The listing builds one solid part. Answer for the finished solid, in the listing's coordinates (mm). A direction names the side the tool comes from. Give positions to 0.01 mm unless a question says otherwise; leave off trailing zeros. Write each loop counter-clockwise with the first axis right and the second up, starting at its lowest first coordinate (ties: lowest second). Pieces come first, ordered by that corner, then holes. Notation, with made-up numbers: (30, 14.25) - (35, 14.25) arc R28 ccw to (35, 47.25) - close; hole circle Ø2 at (48.5, 51.5). An arc over 180 degrees is marked (long way). Answer as CSV lines item,"result". Start each with the question number.
(1) Straight lines are drawn through the part: probe 1 along X at (y, z) = (4, -1.5); probe 2 along Y at (x, z) = (-26, 8); probe 3 along X at (y, z) = (9.5, 3.25). For each, find the intervals that lie inside material, in ascending order.
(2) Find section C-C (z = 5.25). Write down the section's boundary in (x, y).
(3) Each of these flat-tipped pins is pushed along its axis until it touches: pin 1 Ø0.9 at (x, z) = (-18, 2) entering from -Y; pin 2 Ø6 at (x, y) = (-28, 10.5) entering from -Z; pin 3 Ø6 at (x, y) = (-21.5, 4.5) entering from +Z; pin 4 Ø8 at (x, z) = (-29.5, 10) entering from -Y. Where does it stop, or does it pass through?
(4) Find section D-D (y = 11.25). Write down the section's boundary in (x, z).
(5) Find section A-A (y = 3.5). Write down the section's boundary in (x, z).
(6) For a pull along X with two mould halves and no side action, classify faces 4 (the face through (3, 8, -1)), 5 (the face through (-53, 3, -1)), 6 (the face through (0, 6, 8)) as pulls with the +X half, pulls with the -X half, needs draft (parallel to the pull), parting line crosses it, or undercut.
(7) For faces 1 (the face through (-21, 12, -7)), 2 (the face through (-3, 5, 2)), 3 (the face through (-21, 12, 8)), determine the directions among +Z, -Z, +X, -X, +Y, -Y from which every point of the face is accessible in a straight line to the end or side of a thin tool.
(8) Find section B-B (x = -17). Write down the section's boundary in (y, z), then the cut area to 3 significant figures.
from build123d import *

# Parameters (mm, degrees)
PAD_DEPTH         = 3
PAD001_DEPTH      = 10
PAD001_DEPTH_BACK = 18
POCKET_DEPTH      = 5


with BuildPart() as part:
    # Sketch → Pad (new body)
    with BuildSketch(Plane.XY):
        Polygon((-43, 12), (0, 12), (0, 0), (-50, 0), (-50, 4.858572), align=None)
    extrude(amount=PAD_DEPTH)

    # Sketch001 (on Face7 of Pad) → Pad001 (join, two sides)
    with BuildSketch(Plane.XY.offset(3)) as pad001_sk:
        Polygon((-50, 0), (-53, 0), (-53, 6.083674), (-44.260252, 15), (0, 15), (3, 15), (3, 0), (0, 0), (0, 12), (-43, 12), (-50, 4.858572), align=None)
    extrude(amount=PAD001_DEPTH)
    extrude(pad001_sk.sketch, amount=-PAD001_DEPTH_BACK)

    # Sketch002 (on Face18 of Pad001) → Pocket (cut)
    with BuildSketch(Plane.XY.offset(3)):
        Polygon((-48, 0), (-48, 4.041837), (-42.159832, 10), (-3, 10), (-3, 0), align=None)
    extrude(amount=-POCKET_DEPTH, mode=Mode.SUBTRACT)


solid = part.part
Result set:
1,probe 1,"-53 to -50, 0 to 3"
1,probe 2,"12 to 15"
1,probe 3,"-49.65 to -45.45, 0 to 3"
2,outline,"(-53, 0) - (-50, 0) - (-50, 4.86) - (-43, 12) - (0, 12) - (0, 0) - (3, 0) - (3, 15) - (-44.26, 15) - (-53, 6.08) - close"
3,pin 1,"y = 10"
3,pin 2,"z = -15"
3,pin 3,"through"
3,pin 4,"y = 12"
4,outline,"(-47.94, -15) - (-43.74, -15) - (-43.74, 0) - (0, 0) - (0, -15) - (3, -15) - (3, 13) - (0, 13) - (0, 3) - (-43.74, 3) - (-43.74, 13) - (-47.94, 13) - close"
5,outline,"(-53, -15) - (-50, -15) - (-50, 0) - (-48, 0) - (-48, 3) - (-50, 3) - (-50, 13) - (-53, 13) - close; (-3, 0) - (0, 0) - (0, -15) - (3, -15) - (3, 13) - (0, 13) - (0, 3) - (-3, 3) - close"
6,face 4,"pulls with the +X half"
6,face 5,"pulls with the -X half"
6,face 6,"undercut"
7,face 1,"-Z, -Y"
7,face 2,"+Z, -Z, -Y"
7,face 3,"+Z, -Y"
8,outline,"(10, 0) - (12, 0) - (12, -15) - (15, -15) - (15, 13) - (12, 13) - (12, 3) - (10, 3) - close"
8,area,"90.0 mm^2"
